Check sheet for the modelled part. Datum: model origin and axes. Units: mm. A direction names the side the tool comes from. Round coordinates to 2 decimals unless told otherwise and drop trailing zeros. Write each loop counter-clockwise with the first axis right and the second up, starting at its lowest first coordinate (ties: lowest second). Pieces come first, ordered by that corner, then holes. Notation, with made-up numbers: M -33.75,44.5 L 3.25,44.5 A14 cw 3.25,50.5 Z; hole C -14,57 d1. An arc over 180 degrees is marked long. Put each result on its own line as item: value.
Autodesk Inventor part; units mm, degrees
ref_plane "YZ Plane" through (0, 0, 0) normal (1, 0, 0) x (0, 1, 0)
ref_plane "XZ Plane" through (0, 0, 0) normal (0, 1, 0) x (-1, 0, 0)
ref_plane "XY Plane" through (0, 0, 0) normal (0, 0, 1) x (1, 0, 0)
sketch "Sketch19" plane through (0, 0, 0) normal (1, 0, 0) x (0, 1, 0)
  line L0 (0, 0) -> (0, -23)
  line L1 (0, -23) -> (16.1239, -58.9399)
  line L2 (17, -63.0332) -> (17, -88.0332)
  line L3 (17, -88.0332) -> (23.5, -88.0332)
  line L4 (23.5, -88.0332) -> (23.5, -63.0332)
  line L5 (22.6239, -58.9399) -> (6.5, -23)
  line L6 (6.5, -23) -> (6.5, 0)
  line L7 (6.5, 0) -> (0, 0)
  arc A0 (17, -63.0332) -> (16.1239, -58.9399) centre (7, -63.0332) ccw
  arc A1 (23.5, -63.0332) -> (22.6239, -58.9399) centre (13.5, -63.0332) ccw
  point P0 (23.2785, -60.9402)
  dimension "d79" = 10
  dimension "d80" = 10
  dimension "d82" = 6.5
  dimension "d83" = 17
  dimension "d84" = 25
  dimension "d85" = 23
  dimension "d86" = 37.9402
extrude "Extrusion7" add sketch "Sketch19" along normal blind 12
sketch "Sketch20" plane through (0, 6.5, 0) normal (0, 1, 0) x (1, 0, 0)
  circle A0 centre (6, 6) radius 6
  line L0 (0, 0) -> (12, 0)
  line L1 (0, 0) -> (12, 0)
  line L2 (0, 0) -> (0, 6)
  line L3 (0, 0) -> (0, 23)
  line L4 (12, 0) -> (12, 6)
  point P0 (6, 0)
  point P1 (6, 0)
  dimension "d89" = 12
extrude "Extrusion8" cut sketch "Sketch20" against normal blind 12 contours L4 L0 A0 | A0 L0 L2
sketch "Sketch21" plane through (0, 23.5, -63.0332) normal (0, 1, 0) x (1, 0, 0)
  circle A0 centre (6, 21) radius 4
  line L0 (0, 25) -> (12, 25)
  arc A1 (0, -57.0332) -> (12, -57.0332) centre (6, -57.0332) ccw
  line L1 (12, -40.0332) -> (12, -57.0332)
  line L2 (0, -40.0332) -> (12, -40.0332)
  line L3 (0, -40.0332) -> (0, -57.0332)
  line L4 (0, -40.0332) -> (2.0021, 21.1309)
  line L5 (12, -40.0332) -> (12, -4.0933)
  line L6 (12, -40.0332) -> (9.9979, 21.1309)
  line L7 (0, 25) -> (0, 0)
  line L8 (0, -40.0332) -> (0, 25)
  line L9 (0, 25) -> (6, 25)
  line L10 (6, 25) -> (12, 25)
  line L11 (12, 0) -> (12, 25)
  line L12 (12, 25) -> (12, -40.0332)
  point P0 (0, -63.0332)
  point P1 (12, -4.0933)
  point P2 (12, 0)
  dimension "d93" = 8
extrude "Extrusion9" cut sketch "Sketch21" against normal up to surface (23.5 mm away) contours A0 L0 L11 L12 L5 L6 | L4 L8 L7 L0 A0
sketch "Sketch22" plane through (6, 6.5, -6) normal (0, 1, 0) x (1, 0, 0)
  arc A0 (-6, 0) -> (6, 0) centre (0, 0) ccw
  point P0 (-6, -6)
hole "Hole1" at (6, 6.5, -6) direction (0, -1, 0) diameter 10 end through all
sketch "Sketch23" plane through (6, 23.5, -84.0332) normal (0, 1, 0) x (1, 0, 0)
  arc A0 (3.9979, 0.1309) -> (-3.9979, 0.1309) centre (0, 0) ccw
  point P0 (-6, -84.0332)
hole "Hole2" at (6, 23.5, -84.0332) direction (0, -1, 0) diameter 5 end through all
fillet "Fillet1" radius 10 1 edges at (6, 6.5, -23)
properties part number "47B"
1. Cross-section at B-B (y = 5.5). Enter the section's corners in (x, z), then the cut area to 3 significant figures.
Computed values:
outline: M 0,-23 L 0.4,-35.26 L 11.6,-35.26 L 12,-23 L 12,-6 A6 ccw 0,-6 Z; hole C 6,-6 d10
area: 324 mm2
2. Cross-section at C-C (y = 1.5). Enter the section's corners in (x, z).
Computed values:
outline: M 0,-23 L 0.11,-26.34 L 11.89,-26.34 L 12,-23 L 12,-6 A6 ccw 0,-6 Z; hole C 6,-6 d10
3. Access from +Z, -Z, +X, -X, +Y, -Y to the whole of each face (thin tool, end or side, straight path). Record for faces 4 (the flat face through (6, 17, -73)), 5 (the flat face through (6, 23.5, -73)), 6 (the flat face through (6, 6.5, -13)).
Computed values:
face 4: -Z, +X, -X, -Y
face 5: +Z, -Z, +X, -X, +Y
face 6: +Z, +X, -X, +Y
4. Cross-section at D-D (z = -66). Enter the section's corners in (x, y), then the cut area to 3 significant figures.
Computed values:
outline: M 1.41,17 L 10.59,17 L 10.59,23.5 L 1.41,23.5 Z
area: 59.7 mm2
5. Release check for a two-part mould opening along X. For faces 1 (the cylindrical face through (5.25, 20.2, -81.65)), 2 (the cylindrical face through (6.086, 20.296, -88.032)), 3 (the cylindrical face through (5.93, 16.77, -60.91)) record: +X half, -X half, draft (parallel to the pull), parting line (faces both ways), or undercut.
Computed values:
face 1: undercut
face 2: parting line
face 3: draft
6. Depth check by flat-ended pin: pin 1 Ø3 at (x, z) = (3.5, -81.5) entering from -Y; pin 2 Ø5 at (x, z) = (5.5, -27) entering from +Y; pin 3 Ø5 at (x, y) = (6.5, 12.5) entering from +Z. Enter the tip coordinate at first touch or a pass-through.
Computed values:
pin 1: stops at y = 17
pin 2: stops at y = 9.42
pin 3: stops at z = -30.8
7. Cross-section at A-A (x = 6). Enter the section's corners in (y, z), then the cut area to 3 significant figures.
Computed values:
outline: M 0,-23 L 16.12,-58.94 A10 cw 17,-63.03 L 17,-81.53 L 23.5,-81.53 L 23.5,-63.03 A10 ccw 22.62,-58.94 L 7.38,-24.95 A10 cw 6.5,-20.86 L 6.5,-11 L 0,-11 Z; M 0,-1 L 6.5,-1 L 6.5,0 L 0,0 Z; M 17,-88.03 L 23.5,-88.03 L 23.5,-86.53 L 17,-86.53 Z
area: 475 mm2
8. Scan lines: probe 1 along X at (y, z) = (1.5, -6); probe 2 along X at (y, z) = (3.25, -9); probe 3 along Y at (x, z) = (2, -78). Record each from-to range of solid material in increasing order.
Computed values:
probe 1: x = 0 to 1, 11 to 12
probe 2: x = 0 to 2, 10 to 12
probe 3: y = 17 to 23.5
